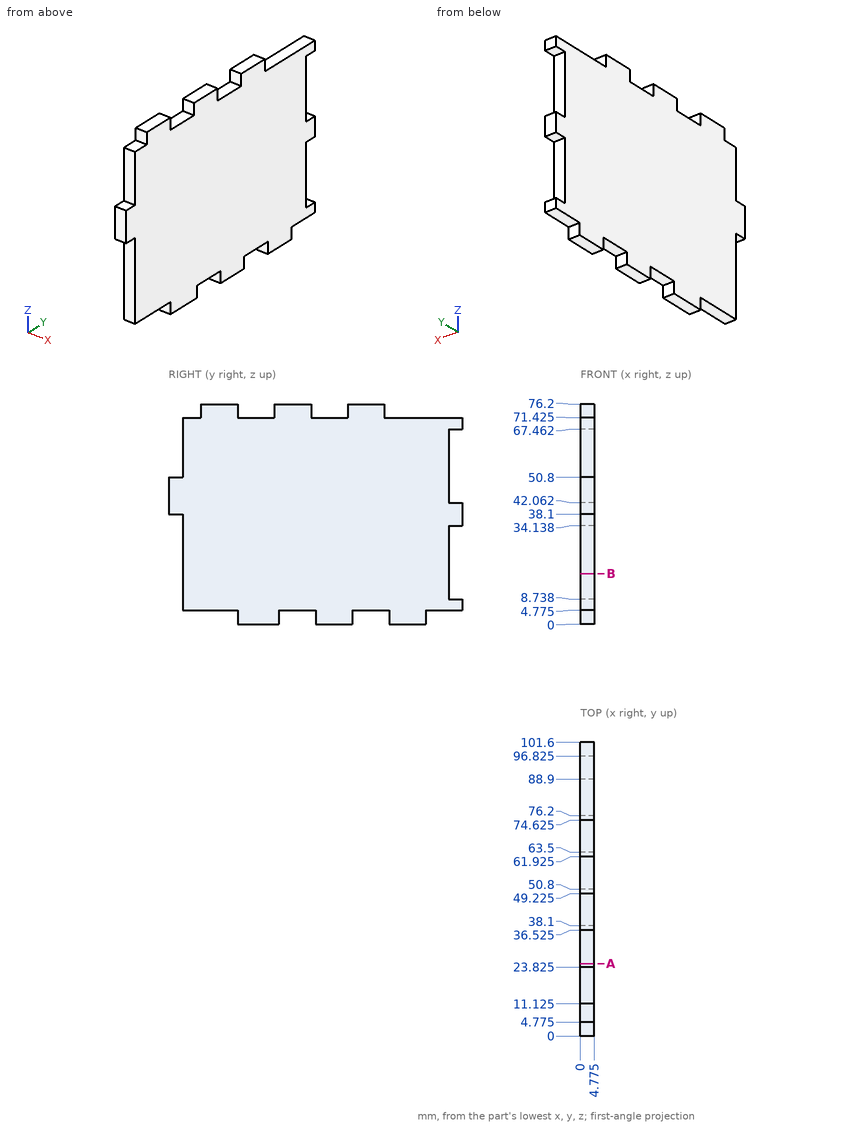
For this review, use the dimensioned drawing (mm, ordinates from the lowest corner) and the shaded views. Give positions to 0.01 mm unless a question says otherwise; leave off trailing zeros. Write each loop counter-clockwise with the first axis right and the second up, starting at its lowest first coordinate (ties: lowest second). Pieces come first, ordered by that corner, then holes. Notation, with made-up numbers: M -22.5,45 L 0.5,45 A34 ccw 0.5,79 Z; hole C 15,25 d7. An arc over 180 degrees is marked long. Answer as a JSON object with one key per item and string values. Group by question number.
Item 1: For probe 1 along Y at (x, z) = (2.5, 73.5) (1 decimal); probe 2 along Y at (x, z) = (2.95, 3.5) (1 decimal); probe 3 along Y at (x, z) = (0.85, 36.5) (1 decimal), list the stretches that pass through material, from the lowest coordinate up. Write a range as [from, to].
Item 2: Consider section A-A on y = 25. Write out the cut boundary in (x, z) (1 decimal).
Item 3: Consider section B-B on z = 17.5. Write out the cut boundary in (x, y) (1 decimal).
Item 4: For pin 1 Ø2.5 at (x, y) = (1.5, 3) entering from +Z; pin 2 Ø1.4 at (x, z) = (3, 56) entering from -Y (1 decimal); pin 3 Ø2.5 at (x, z) = (2.5, 1.5) entering from +Y, all flat-tipped, find the tip position at first contact; note any pin that passes through.
Check result:
{
 "1": {"probe 1": "y = [11.1, 23.8], [36.5, 49.2], [61.9, 74.6]", "probe 2": "y = [23.8, 38.1], [50.8, 63.5], [76.2, 88.9]", "probe 3": "y = [4.8, 101.6]"},
 "2": {"outline": "M 0,0 L 4.8,0 L 4.8,71.4 L 0,71.4 Z"},
 "3": {"outline": "M 0,4.8 L 4.8,4.8 L 4.8,96.8 L 0,96.8 Z"},
 "4": {"pin 1": "stops at z = 50.8", "pin 2": "stops at y = 4.8", "pin 3": "stops at y = 88.9"}
}
